Check sheet for the modelled part. Datum: model origin and axes. Units: mm. Face numbers are marked on the shaded views. A direction names the side the tool comes from. Round coordinates to 2 decimals unless told otherwise and drop trailing zeros. Write each loop counter-clockwise with the first axis right and the second up, starting at its lowest first coordinate (ties: lowest second). Pieces come first, ordered by that corner, then holes.
Item 1: Cross-section at B-B on z = -8.25. Enter the section's corners in (x, y) (3 decimals).
Item 2: Release check for a two-part mould opening along X. For the marked faces 1, 2 and 3 record: +X half, -X half, draft (parallel to the pull), parting line (faces both ways), or undercut.
Item 3: Cross-section at C-C on x = 8.75. Enter the section's corners in (y, z).
Item 4: Tool access check on the marked faces 4, 5 and 6. Record the directions out of +Z, -Z, +X, -X, +Y, -Y that give a thin tool (end or side, any length) a straight path to the whole face; none if there is none.
Item 5: Go/stop test with flat-tipped pins: pin 1 Ø2.5 at (y, z) = (0.5, 1) entering from -X; pin 2 Ø3.5 at (x, z) = (-1.5, -4) entering from +Y; pin 3 Ø1.5 at (y, z) = (1, 7.5) entering from +X. Record where each tip stops, or that it passes through.
Item 6: Cross-section at A-A on y = 2.5. Enter the section's corners in (x, z) (3 decimals).
Item 7: Material ranges on line 1 (X direction, y = 2.5, z = 0.75) (3 decimals); line 2 (X direction, y = 4.75, z = 9) (3 decimals); line 3 (Y direction, x = -3.5, z = 1.25), recorded low to high.
Item 8: Cross-section at D-D on y = -1. Enter the section's corners in (x, z).
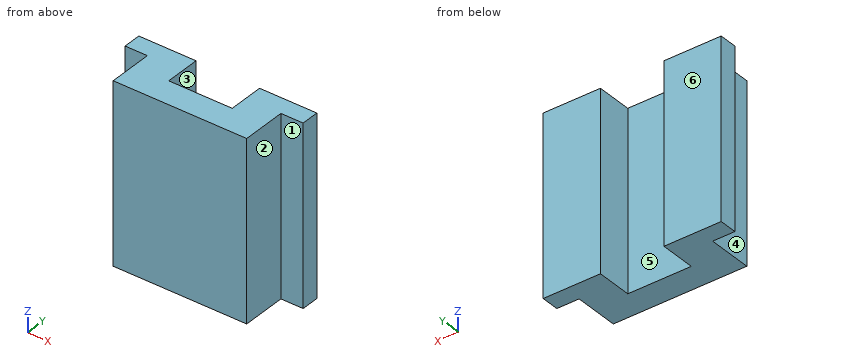
Autodesk Inventor part; units mm, degrees
ref_plane "YZ Plane" through (0, 0, 0) normal (1, 0, 0) x (0, 1, 0)
ref_plane "XZ Plane" through (0, 0, 0) normal (0, 1, 0) x (-1, 0, 0)
ref_plane "XY Plane" through (0, 0, 0) normal (0, 0, 1) x (1, 0, 0)
sketch "Sketch1" plane through (0, 0, 0) normal (0, 1, 0) x (-1, 0, 0)
  line L0 (-10, 10) -> (10, 10)
  line L1 (10, 10) -> (10, -10)
  line L2 (10, -10) -> (-10, -10)
  line L3 (-10, -10) -> (-10, 10)
  line L4 (-10, 10) -> (10, -10) construction
  line L5 (10, 10) -> (-10, -10) construction
  point P0 (0, 0)
  dimension "d0" = 20
  dimension "d1" = 20
extrude "Extrusion1" add sketch "Sketch1" along normal mid plane 3
sketch "Sketch2" plane through (0, 1.5, 0) normal (0, 1, 0) x (1, 0, 0)
  line L0 (-10, -10) -> (10, -10)
  line L1 (10, -10) -> (10, 10)
  line L2 (10, 10) -> (-10, 10)
  line L3 (-10, 10) -> (-10, -10)
  line L4 (-3.565, -10) -> (3.565, -10)
  line L5 (3.565, -10) -> (3.565, 10)
  line L6 (3.565, 10) -> (-3.565, 10)
  line L7 (-3.565, 10) -> (-3.565, -10)
  point P0 (0, 0)
  point P1 (0, 10)
  dimension "d5" = 7.13
extrude "Extrusion2" add sketch "Sketch2" along normal blind 4 contours L3 L2 L7 L0 | L5 L2 L1 L0
sketch "Sketch3" plane through (-10, -1.5, 10) normal (0, 0, 1) x (1, 0, 0)
  line L0 (0, 7) -> (0, 0)
  line L1 (2.5, 5) -> (0, 5)
  line L2 (0, 5) -> (0, 0)
  line L3 (0, 0) -> (2.5, 0)
  line L4 (2.5, 0) -> (2.5, 5)
  line L5 (2.5, 5) -> (0, 0) construction
  line L6 (0, 5) -> (2.5, 0) construction
  line L7 (20, 0) -> (0, 0)
  line L8 (17.5, 5) -> (20, 5)
  line L9 (20, 5) -> (20, 0)
  line L10 (20, 0) -> (17.5, 0)
  line L11 (17.5, 0) -> (17.5, 5)
  line L12 (17.5, 5) -> (20, 0) construction
  line L13 (20, 5) -> (17.5, 0) construction
  point P0 (10, 1.5)
  point P1 (1.25, 2.5)
  point P2 (18.75, 2.5)
  point P3 (1.25, 2.5)
  point P4 (18.75, 2.5)
  dimension "d8" = 2.5
  dimension "d9" = 5
extrude "Extrusion3" cut sketch "Sketch3" against normal through all
properties part number "RS-FixedFiber"
Response values:
1. outline: (-10, 3.5) - (-7.5, 3.5) - (-7.5, -1.5) - (7.5, -1.5) - (7.5, 3.5) - (10, 3.5) - (10, 5.5) - (3.565, 5.5) - (3.565, 1.5) - (-3.565, 1.5) - (-3.565, 5.5) - (-10, 5.5) - close
2. face 1: draft
2. face 2: +X half
2. face 3: undercut
3. outline: (3.5, -10) - (5.5, -10) - (5.5, 10) - (3.5, 10) - close
4. face 4: +Z, -Z, -X, -Y
4. face 5: +Z, -Z, +Y
4. face 6: +Z, -Z, +X, -X, +Y
5. pin 1: stops at x = -7.5
5. pin 2: stops at y = 1.5
5. pin 3: stops at x = 7.5
6. outline: (-7.5, -10) - (-3.565, -10) - (-3.565, 10) - (-7.5, 10) - close; (3.565, -10) - (7.5, -10) - (7.5, 10) - (3.565, 10) - close
7. line 1: x = -7.5 to -3.565, 3.565 to 7.5
7. line 2: x = -10 to -3.565, 3.565 to 10
7. line 3: y = -1.5 to 1.5
8. outline: (-7.5, -10) - (7.5, -10) - (7.5, 10) - (-7.5, 10) - close
